```python
from build123d import *

# Parameters (mm, degrees)
SKETCH1_R           = 2.54
BOSS_EXTRUDE1_DEPTH = 5.08
SKETCH1_2_R         = 2.54
BOSS_EXTRUDE2_DEPTH = 1.016


with BuildPart() as part:
    # Sketch1 → Boss-Extrude1 (new body)
    with BuildSketch(Plane(origin=(0, 0, 0), x_dir=(0, 0, -1), z_dir=(1, 0, 0))):
        with BuildLine():
            Line((-3.81, 0), (-2.507191408, -8.026929038))
            ThreePointArc((-2.507191408, -8.026929038), (0, -10.16), (2.507191408, -8.026929038))
            Line((2.507191408, -8.026929038), (3.81, 0))
            ThreePointArc((3.81, 0), (0, 3.81), (-3.81, 0))
        make_face()
        Circle(SKETCH1_R, mode=Mode.SUBTRACT)
    extrude(amount=BOSS_EXTRUDE1_DEPTH)

    # Sketch1<2> → Boss-Extrude2 (add)
    with BuildSketch(Plane(origin=(0, 0, 0), x_dir=(0, 0, -1), z_dir=(1, 0, 0))):
        Circle(SKETCH1_2_R)
    extrude(amount=BOSS_EXTRUDE2_DEPTH)


solid = part.part
```
Geometry: final body of the model. Coordinates: model frame, mm. A direction names the side the tool comes from. Coordinates: 2 decimals unless noted, no trailing zeros. Order: outer loops, then holes, each group sorted by start corner. A loop starts at its lowest first (then second) coordinate and runs counter-clockwise, first axis right, second up. Notation, with made-up numbers: (-32.75, -25) - (-27.75, -25) arc R37 ccw to (-27.75, 13) - close; hole circle Ø6 at (81.25, 68). An arc over 180 degrees is marked (long way). Return JSON: item names as keys, results as strings. Group by question number.
1. Set-up query: faces 4 (the face through (3.02, 2.52, 0.33)), 5 (the face through (2.5, -4.07, -3.15)). Return all of +Z, -Z, +X, -X, +Y, -Y with unobstructed straight access to the full face (end or side cutting, diameter ignored); none if empty.
2. Cut plane C-C (y = -1). Output: boundary loops of the cut face in (x, z).
3. Cut plane B-B (z = 0). Output: boundary loops of the cut face in (x, y).
4. Cut plane D-D (z = 3.25). Output: boundary loops of the cut face in (x, y).
5. Cut plane A-A (x = 3). Output: boundary loops of the cut face in (y, z).
6. Material intervals for line 1 along X through (y, z) = (1.5, 1.75); line 2 along Y through (x, z) = (3.25, -1.5); line 3 along Z through (x, y) = (4, -1.75), sorted ascending. Write a range as [from, to].
7. Pull-direction query (Y, two-part tool) for faces 1 (the face through (2.504, -3.957, 3.168)), 2 (the face through (5.08, -3, 0)), 3 (the face through (1.016, 0, 0)); classes: pulls with the +Y half, pulls with the -Y half, needs draft (parallel to the pull), parting line crosses it, or undercut.
8. Pin query (flat end, axial travel): pin 1 (3 mm diameter, centred on x = 1, y = -7, fed in from -Z). Return the tip coordinate at first contact, or that it passes through.
Resolved:
{
 "1": {"face 4": "+X", "face 5": "-Z, +X, -X, -Y"},
 "2": {"outline": "(0, -3.65) - (5.08, -3.65) - (5.08, -2.33) - (1.02, -2.33) - (1.02, 2.33) - (5.08, 2.33) - (5.08, 3.65) - (0, 3.65) - close"},
 "3": {"outline": "(0, -10.16) - (5.08, -10.16) - (5.08, -2.54) - (1.02, -2.54) - (1.02, 2.54) - (5.08, 2.54) - (5.08, 3.81) - (0, 3.81) - close"},
 "4": {"outline": "(0, -3.45) - (5.08, -3.45) - (5.08, 1.99) - (0, 1.99) - close"},
 "5": {"outline": "(-8.03, -2.51) - (0, -3.81) arc R3.81 ccw to (0, 3.81) - (-8.03, 2.51) arc R2.54 ccw to start; hole circle Ø5.08 at (0, 0)"},
 "6": {"line 1": "x = [0, 1.02]", "line 2": "y = [-9.67, -2.05], [2.05, 3.5]", "line 3": "z = [-3.53, -1.84], [1.84, 3.53]"},
 "7": {"face 1": "pulls with the -Y half", "face 2": "needs draft", "face 3": "undercut"},
 "8": {"pin 1": "stops at z = -2.92"}
}
